Input: part model. Units: mm. Frame: model coordinates. A direction names the side the tool comes from. Coordinates: 2 decimals unless noted, no trailing zeros. Order: outer loops, then holes, each group sorted by start corner. A loop starts at its lowest first (then second) coordinate and runs counter-clockwise, first axis right, second up. Notation, with made-up numbers: (2, 47) -> (22, 47) arc R13 ccw to (22, 62) -> close; hole circle Ø3 at (-23, 50). An arc over 180 degrees is marked (long way). Use CSV: the item, a comma, the result in double quotes. Start each with the question number.
```python
from build123d import *

# Parameters (mm, degrees)
F0_R     = 3.7338
F1_DEPTH = 1.8034
F2_R     = 2.2606
F3_DEPTH = 5.9182
F4_R     = 2.2606
F5_DEPTH = 5.9182
F6_R     = 1.0414
F7_DEPTH = 25.4


with BuildPart() as f1:
    # F0 (on Top) → F1 (new body)
    with BuildSketch(Plane.XY):
        Circle(F0_R)
    extrude(amount=F1_DEPTH)

    # F2 (on face) → F3 (join)
    with BuildSketch(Plane.XY.offset(1.8034)):
        Circle(F2_R)
    extrude(amount=F3_DEPTH)

    # F4 (on face) → F5 (join)
    with BuildSketch(Plane(origin=(0, 0, 0), x_dir=(1, 0, 0), z_dir=(0, 0, -1))):
        Circle(F4_R)
    extrude(amount=F5_DEPTH)

    # F6 (on face) → F7 (cut)
    with BuildSketch(Plane(origin=(0, 0, -5.9182), x_dir=(1, 0, 0), z_dir=(0, 0, -1))):
        Circle(F6_R)
    extrude(amount=-F7_DEPTH, mode=Mode.SUBTRACT)


solid = f1.part
```
1. Section D-D on z = 1.25. Return loops of the section in (x, y), then the cut area to 3 significant figures.
2. Section C-C on z = 3.5. Return loops of the section in (x, y).
3. Section A-A on x = 0. Return loops of the section in (y, z), then the cut area to 3 significant figures.
4. Contact query for flat-ended pins moving along their axis: P1, Ø1, axis at y = 1.5, z = 3, coming from the +X side; P2, Ø1.5, axis at y = 1, z = -1, coming from the -X side; P3, Ø1.2, axis at x = 0, y = 0, coming from the -Z side. Output: stop coordinate, or through.
5. Material intervals for line 1 along Y through (x, z) = (0, -2); line 2 along Y through (x, z) = (0, 1.5); line 3 along Z through (x, y) = (2.5, -1), sorted ascending.
6. Access query for faces 1 (the face through (2, -2, 1.803)), 2 (the face through (1, 1, 7.722)), 3 (the face through (2, -2, 0)). Directions: +Z, -Z, +X, -X, +Y, -Y. A direction counts if a zero-diameter tool reaches every point of the face in a straight line with its end or side. Return the directions, or none.
7. Section B-B on y = 0.75. Return loops of the section in (x, z).
8. Pull-direction query (Y, two-part tool) for faces 4 (the face through (-0.49, -2.207, 4.721)), 5 (the face through (0.993, -0.313, 0.806)), 6 (the face through (1, -1, -5.918)); classes: released by +Y, released by -Y, zero draft, split by the parting line, or undercut.
Values follow:
1,outline,"circle Ø7.47 at (0, 0); hole circle Ø2.08 at (0, 0)"
1,area,"40.4 mm2"
2,outline,"circle Ø4.52 at (0, 0); hole circle Ø2.08 at (0, 0)"
3,outline,"(-3.73, 0) -> (-2.26, 0) -> (-2.26, -5.92) -> (-1.04, -5.92) -> (-1.04, 7.72) -> (-2.26, 7.72) -> (-2.26, 1.8) -> (-3.73, 1.8) -> close; (1.04, -5.92) -> (2.26, -5.92) -> (2.26, 0) -> (3.73, 0) -> (3.73, 1.8) -> (2.26, 1.8) -> (2.26, 7.72) -> (1.04, 7.72) -> close"
3,area,"38.6 mm2"
4,P1,"stops at x = 2.03"
4,P2,"stops at x = -2.25"
4,P3,"passes through"
5,line 1,"y = -2.26 to -1.04, 1.04 to 2.26"
5,line 2,"y = -3.73 to -1.04, 1.04 to 3.73"
5,line 3,"z = 0 to 1.8"
6,face 1,"+Z"
6,face 2,"+Z, +X, -X, +Y, -Y"
6,face 3,"-Z"
7,outline,"(-3.66, 0) -> (-2.13, 0) -> (-2.13, -5.92) -> (-0.72, -5.92) -> (-0.72, 7.72) -> (-2.13, 7.72) -> (-2.13, 1.8) -> (-3.66, 1.8) -> close; (0.72, -5.92) -> (2.13, -5.92) -> (2.13, 0) -> (3.66, 0) -> (3.66, 1.8) -> (2.13, 1.8) -> (2.13, 7.72) -> (0.72, 7.72) -> close"
8,face 4,"split by the parting line"
8,face 5,"undercut"
8,face 6,"zero draft"
